```python
from build123d import *

# Parameters (mm, degrees)
SKETCH_1_W               = 10
SKETCH_1_H               = 20
SKETCH_1_W_2             = 15
SKETCH_1_H_2             = 19
SKETCH_1_W_3             = 7.75
SKETCH_1_H_3             = 3
EXTRUDE_1_DEPTH          = 3
CUT_EXTRUDE_1_DEPTH      = 70.392002421
CUT_EXTRUDE_1_DEPTH_BACK = 70.392002421
SKETCH_2_R               = 2


with BuildPart() as part:
    # 草图1 → 凸台-拉伸1 (new body)
    with BuildSketch(Plane.XY):
        with Locations((-20, -49.5)):
            Rectangle(SKETCH_1_W, SKETCH_1_H)
        with Locations((22.5, -50)):
            Rectangle(SKETCH_1_W_2, SKETCH_1_H_2)
        Polygon((-2.25, 58.5), (-2.25, 59.5), (-10, 59.5), (-15, 59.5), (-15, -39.5), (-15, -59.5), (15, -59.5), (15, -40.5), (15, 59.5), (10, 59.5), (2.25, 59.5), (2.25, 58.5), (4.25, 58.5), (4.25, 53.5), (2.25, 53.5), (2.25, 47.5), (-2.25, 47.5), (-2.25, 53.5), (-4.25, 53.5), (-4.25, 58.5), align=None)
        with Locations((6.125, 61)):
            Rectangle(SKETCH_1_W_3, SKETCH_1_H_3)
        with Locations((-6.125, 61)):
            Rectangle(SKETCH_1_W_3, SKETCH_1_H_3)
    extrude(amount=EXTRUDE_1_DEPTH)

    # 草图2 → 切除-拉伸1 (cut, two sides: drawn at the far end of the back side and taken through both)
    with BuildSketch(Plane.XY.offset(3).offset(-CUT_EXTRUDE_1_DEPTH_BACK)):
        with Locations((-9.288837026, -50.295936885)):
            Circle(SKETCH_2_R)
        with Locations((10.711162974, -50.295936885)):
            Circle(SKETCH_2_R)
    extrude(amount=CUT_EXTRUDE_1_DEPTH + CUT_EXTRUDE_1_DEPTH_BACK, mode=Mode.SUBTRACT)


solid = part.part
```
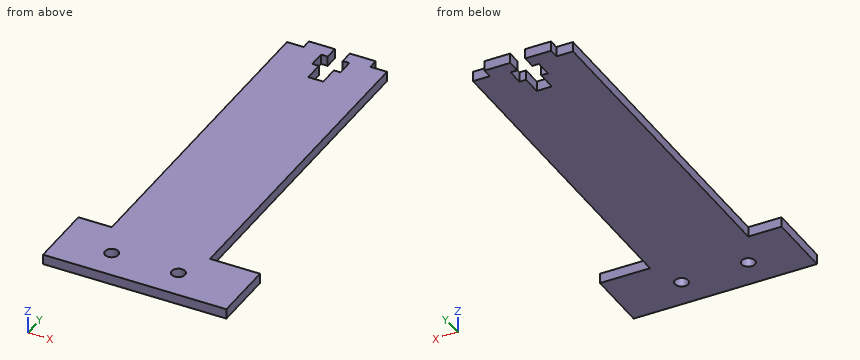
The model under review builds one solid part; all positions refer to its coordinate system, in mm. Round coordinates to 2 decimals unless told otherwise and drop trailing zeros. Loops run counter-clockwise (first coordinate to the right, second up) from the corner with the lowest first, then second, coordinate; pieces in that order, holes last. Notation, with made-up numbers: (25, 57.25) - (59, 57.25) arc R18 ccw to (59, 85.25) - close; hole circle Ø9 at (27, 13.25). An arc over 180 degrees is marked (long way). Use a Markdown table: item, result. Add a question column.
Q1. Add section C-C (x = 18.5). State the section outline as (y, z) points, plus the area to 3 significant figures.
Q2. Add section A-A (z = 2.3). State the section outline as (x, y) points, plus the area to 3 significant figures.
Q3. Add section B-B (y = 0). State the section outline as (x, z) points.
Q4. For probe 1 along Y at (x, z) = (-9.5, 0.25); probe 2 along X at (y, z) = (38.5, 2.55); probe 3 along Y at (x, z) = (19, 0.65), list the stretches that pass through material, from the lowest coordinate up.
Q5. Insertion check: pin 1 Ø0.9 at (x, z) = (-0.5, 2) entering from +Y; pin 2 Ø1.5 at (y, z) = (-2.5, 0.5) entering from +X; pin 3 Ø0.9 at (y, z) = (49.5, 1.5) entering from -X. Each pin has a flat end and moves straight along its axis. Give the tip position at first contact, or say it passes through.
Worked answers:
| question | item | result |
|---|---|---|
| 1 | outline | (-59.5, 0) - (-40.5, 0) - (-40.5, 3) - (-59.5, 3) - close |
| 1 | area | 57.0 mm² |
| 2 | outline | (-25, -59.5) - (30, -59.5) - (30, -40.5) - (15, -40.5) - (15, 59.5) - (10, 59.5) - (10, 62.5) - (2.25, 62.5) - (2.25, 58.5) - (4.25, 58.5) - (4.25, 53.5) - (2.25, 53.5) - (2.25, 47.5) - (-2.25, 47.5) - (-2.25, 53.5) - (-4.25, 53.5) - (-4.25, 58.5) - (-2.25, 58.5) - (-2.25, 62.5) - (-10, 62.5) - (-10, 59.5) - (-15, 59.5) - (-15, -39.5) - (-25, -39.5) - close; hole circle Ø4 at (-9.29, -50.3); hole circle Ø4 at (10.71, -50.3) |
| 2 | area | 4,000 mm² |
| 3 | outline | (-15, 0) - (15, 0) - (15, 3) - (-15, 3) - close |
| 4 | probe 1 | -59.5 to -52.28, -48.31 to 62.5 |
| 4 | probe 2 | -15 to 15 |
| 4 | probe 3 | -59.5 to -40.5 |
| 5 | pin 1 | y = 47.5 |
| 5 | pin 2 | x = 15 |
| 5 | pin 3 | x = -15 |
